Check sheet for the modelled part. Datum: model origin and axes. Units: mm. Coordinates: 2 decimals unless noted, no trailing zeros. Write each loop counter-clockwise with the first axis right and the second up, starting at its lowest first coordinate (ties: lowest second). Pieces come first, ordered by that corner, then holes. Notation, with made-up numbers: (-21, -14.75) -> (16, -14.75) arc R11 cw to (16, -9.75) -> close; hole circle Ø4 at (25.25, 22.25). An arc over 180 degrees is marked (long way). One line per item, written item: value. Start each with the question number.
1) Sectioned sample at B-B on z = 207. Enter the section's corners in (x, y), plus the area to 3 significant figures.
2) Sectioned sample at D-D on z = 240.5. Enter the section's corners in (x, y).
3) Scan lines: line 1 along X through (y, z) = (9.75, 225.5); line 2 along X through (y, z) = (4, 193); line 3 along X through (y, z) = (3.25, 235.5). Record each from-to range of solid material in increasing order. Write a range as [from, to].
4) Gauge pin test, flat end, axial feed: P1, Ø6, axis at y = 5.5, z = 272.5, coming from the -X side. Record the tip position at first contact, or that the pin passes through.
5) Sectioned sample at A-A on x = -132.5. Enter the section's corners in (y, z).
6) Sectioned sample at C-C on y = 6. Enter the section's corners in (x, z).
```python
from build123d import *

# Parameters (mm, degrees)
F1_DEPTH = 10
F2_DEPTH = 25
F3_DEPTH = 25


with BuildPart() as f1:
    # F0 (on Front) → F1 (new body)
    with BuildSketch(Plane.XZ):
        with BuildLine():
            ThreePointArc((-120, 235), (-139.038059, 280.961941), (-185, 300))
            ThreePointArc((-185, 300), (-230.961941, 280.961941), (-250, 235))
            ThreePointArc((-250, 235), (-185, 170), (-120, 235))
        make_face()
        with BuildLine():
            Line((0, 300), (-185, 300))
            ThreePointArc((-185, 300), (-139.038059, 280.961941), (-120, 235))
            ThreePointArc((-120, 235), (-185, 170), (-250, 235))
            Line((-250, 235), (-250, 160))
            Line((-250, 160), (0, 160))
            Line((0, 160), (0, 300))
        make_face()
        with BuildLine():
            Line((185, 300), (0, 300))
            Line((0, 300), (0, 160))
            Line((0, 160), (250, 160))
            Line((250, 160), (250, 235))
            ThreePointArc((250, 235), (139.038059, 189.038059), (185, 300))
        make_face()
        with BuildLine():
            ThreePointArc((250, 235), (230.961941, 280.961941), (185, 300))
            ThreePointArc((185, 300), (139.038059, 189.038059), (250, 235))
        make_face()
    extrude(amount=-F1_DEPTH)

    # F0 (on Front) → F2 (cut)
    with BuildSketch(Plane.XZ):
        with BuildLine():
            ThreePointArc((-120, 235), (-139.038059, 280.961941), (-185, 300))
            ThreePointArc((-185, 300), (-230.961941, 280.961941), (-250, 235))
            ThreePointArc((-250, 235), (-185, 170), (-120, 235))
        make_face()
    extrude(amount=-F2_DEPTH, mode=Mode.SUBTRACT)

    # F0 (on Front) → F3 (cut)
    with BuildSketch(Plane.XZ):
        with BuildLine():
            ThreePointArc((250, 235), (230.961941, 280.961941), (185, 300))
            ThreePointArc((185, 300), (139.038059, 189.038059), (250, 235))
        make_face()
    extrude(amount=-F3_DEPTH, mode=Mode.SUBTRACT)


solid = f1.part
```
Answers:
1. outline: (-250, 0) -> (-243.66, 0) -> (-243.66, 10) -> (-250, 10) -> close; (-126.34, 0) -> (126.34, 0) -> (126.34, 10) -> (-126.34, 10) -> close; (243.66, 0) -> (250, 0) -> (250, 10) -> (243.66, 10) -> close
1. area: 2,650 mm2
2. outline: (-120.23, 0) -> (120.23, 0) -> (120.23, 10) -> (-120.23, 10) -> close
3. line 1: x = [-250, -249.3], [-120.7, 120.7], [249.3, 250]
3. line 2: x = [-250, -234.61], [-135.39, 135.39], [234.61, 250]
3. line 3: x = [-120, 120]
4. P1: stops at x = -134.16
5. outline: (0, 160) -> (10, 160) -> (10, 196.68) -> (0, 196.68) -> close; (0, 273.32) -> (10, 273.32) -> (10, 300) -> (0, 300) -> close
6. outline: (-250, 160) -> (250, 160) -> (250, 235) arc R65 cw (long way) to (185, 300) -> (-185, 300) arc R65 cw (long way) to (-250, 235) -> close
